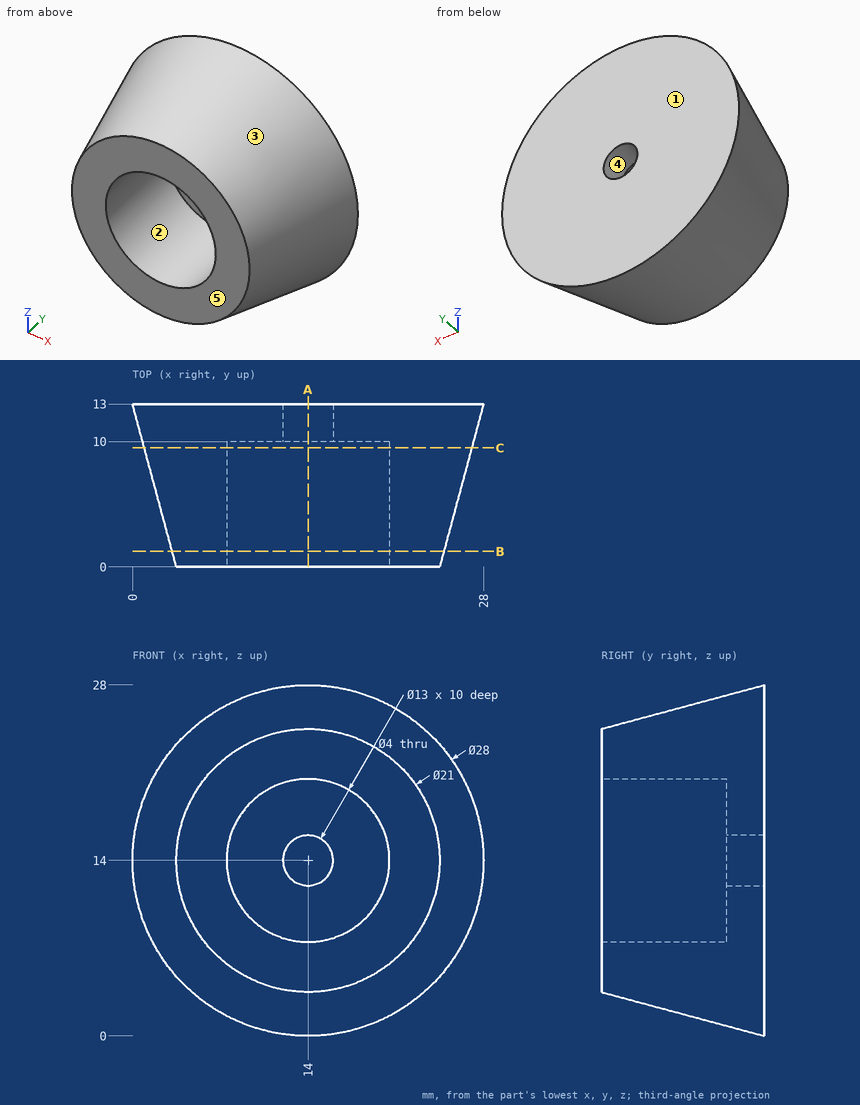
Source: three-view drawing plus pictorial views. Frame: mm from the lowest corner of the part. A direction names the side the tool comes from. Give positions to 0.01 mm unless a question says otherwise; leave off trailing zeros. Write each loop counter-clockwise with the first axis right and the second up, starting at its lowest first coordinate (ties: lowest second). Pieces come first, ordered by that corner, then holes. Notation, with made-up numbers: (9.5, 14) -> (65.5, 14) arc R19 ccw to (65.5, 36) -> close; hole circle Ø6 at (16, 73.5). An arc over 180 degrees is marked (long way). Write item = value, one per line.
Q1. Reachability of the marked faces 1 and 2 from +Z, -Z, +X, -X, +Y, -Y: full face, straight path, thin tool, end or side. Return the list, or none.
Here are the results:
face_1 = +Z, -Z, +X, -X, +Y
face_2 = -Y
Q2. Line query: line 1 (X direction, y = 5.5, z = 14.5); line 2 (Z direction, x = 12, y = 8.75); line 3 (X direction, y = 3.75, z = 11.5). Output: solid intervals per line, ascending. Write a range as from..to.
Here are the results:
line_1 = 2.03..7.52, 20.48..25.97
line_2 = 1.3..7.82, 20.18..26.7
line_3 = 2.77..8, 20..25.23
Q3. Mould query, pull axis X, two halves, no side actions, for the marked faces 3, 4 and 5. Classes: +X half, -X half, draft (parallel to the pull), parting line (faces both ways), or undercut.
Here are the results:
face_3 = parting line
face_4 = undercut
face_5 = draft
Q4. Cut plane C-C on y = 9.5. Return loops of the section in (x, z).
Here are the results:
outline = circle Ø26.12 at (14, 14); hole circle Ø13 at (14, 14)
Q5. Cut plane B-B on y = 1.25. Return loops of the section in (x, z).
Here are the results:
outline = circle Ø21.67 at (14, 14); hole circle Ø13 at (14, 14)
Q6. First-contact query: pin 1 (1 mm diameter, centred on y = 7.5, z = 23.5, fed in from -X); pin 2 (4 mm diameter, centred on y = 7.5, z = 5.5, fed in from -X). Flat tips, straight axial feed; report the tip coordinate or a pass-through.
Here are the results:
pin_1 = 5.26
pin_2 = 3.15
Q7. Cut plane A-A on x = 14. Return loops of the section in (y, z), then the cut area to 4 significant figures.
Here are the results:
outline = (0, 3.5) -> (13, 0) -> (13, 12) -> (10, 12) -> (10, 7.5) -> (0, 7.5) -> close; (0, 20.5) -> (10, 20.5) -> (10, 16) -> (13, 16) -> (13, 28) -> (0, 24.5) -> close
area = 176.5 mm²
